```python
from build123d import *

# Parameters (mm, degrees)
EXTRUDE_1_DEPTH = 5.5
SKETCH_5_R      = 4
EXTRUDE_2_DEPTH = 45
CHAMFER_1_SIZE  = 1


with BuildPart() as part:
    # Эскиз1 → Вытянуть1 (new body)
    with BuildSketch(Plane(origin=(0, 0, 0), x_dir=(1, 0, 0), z_dir=(0, 1, 0))):
        Polygon((-3.75277675, 6.5), (3.75277675, 6.5), (7.505553499, 0), (3.75277675, -6.5), (-3.75277675, -6.5), (-7.505553499, 0), align=None)
    extrude(amount=-EXTRUDE_1_DEPTH)

    # Эскиз5 → Вытянуть2 (add)
    with BuildSketch(Plane.XZ.offset(5.5)):
        with Locations(Location((0, 0, 0), (0, 0, 90))):
            Circle(SKETCH_5_R)
    extrude(amount=EXTRUDE_2_DEPTH)

    # Фаска1
    chamfer_1_edges = [part.edges().sort_by_distance(p)[0] for p in [
        (0, -50.5, -4),
    ]]
    chamfer(chamfer_1_edges, length=CHAMFER_1_SIZE)

    # Эскиз4 → Вырез-Повернуть1 (revolve, cut)
    with BuildSketch(Plane.XY):
        Polygon((-7.505553499, -1), (-6.505553499, 0), (-7.505553499, 0), align=None)
        Polygon((-7.505553499, -4.5), (-6.505553499, -5.5), (-7.505553499, -5.5), align=None)
    revolve(axis=Axis((0, -5.5, 0), (0, -1, 0)), mode=Mode.SUBTRACT)


solid = part.part
```
Input: part model. Units: mm. Frame: model coordinates. A direction names the side the tool comes from. Coordinates: 2 decimals unless noted, no trailing zeros. Loops run counter-clockwise (first coordinate to the right, second up) from the corner with the lowest first, then second, coordinate; pieces in that order, holes last. Notation, with made-up numbers: (-28.5, 8) - (4.5, 8) arc R14 cw to (4.5, 23) - close; hole circle Ø1 at (41.25, 13.25). An arc over 180 degrees is marked (long way). Answer in a Markdown table with one row per item.
(1) Cut plane A-A on y = -29. Output: boundary loops of the cut face in (x, z).
Model answer:
| item | result |
|---|---|
| outline | circle Ø8 at (0, 0) |
(2) Set-up query: faces 1 (the face through (3.377, -5.225, -5.88)), 2 (the face through (3.905, -27.192, -0.867)). Return all of +Z, -Z, +X, -X, +Y, -Y with unobstructed straight access to the full face (end or side cutting, diameter ignored); none if empty.
Model answer:
| item | result |
|---|---|
| face 1 | -Z, +X, -Y |
| face 2 | -Y |
(3) Pin query (flat end, axial travel): P1, Ø1, axis at x = -1, z = 4, coming from the +Y side; P2, Ø4, axis at y = -28.5, z = -3.5, coming from the -X side; P3, Ø8, axis at x = 2.5, y = -28, coming from the +Z side; P4, Ø1.5, axis at y = -37.5, z = 0.5, coming from the -X side. Return the tip coordinate at first contact, or that it passes through.
Model answer:
| item | result |
|---|---|
| P1 | stops at y = 0 |
| P2 | stops at x = -3.71 |
| P3 | stops at z = 4 |
| P4 | stops at x = -4 |
(4) Material intervals for L1, parallel to Y at x = 0.75, z = -5; L2, parallel to Z at x = -2.5, y = -35; L3, parallel to X at y = -26.5, z = -1.75, sorted ascending. Write a range as from..to.
Model answer:
| item | result |
|---|---|
| L1 | y = -5.5..0 |
| L2 | z = -3.12..3.12 |
| L3 | x = -3.6..3.6 |
